from build123d import *

# Parameters (mm, degrees)
SKETCH1_W           = 15
SKETCH1_H           = 49
SKETCH1_R           = 1.6
BOSS_EXTRUDE1_DEPTH = 15
SKETCH2_R           = 2.6
CUT_EXTRUDE1_DEPTH  = 54.394756297
SKETCH5_W           = 15
SKETCH5_H           = 46
BOSS_EXTRUDE3_DEPTH = 10
SKETCH6_R           = 2.6
CUT_EXTRUDE2_DEPTH  = 51.655700568


with BuildPart() as part:
    # Sketch1 → Boss-Extrude1 (new body)
    with BuildSketch(Plane(origin=(0, 0, 0), x_dir=(0, 0, -1), z_dir=(1, 0, 0))):
        with Locations((-7.5, 24.5)):
            Rectangle(SKETCH1_W, SKETCH1_H)
        with Locations((-11, 39.6)):
            Circle(SKETCH1_R, mode=Mode.SUBTRACT)
        with Locations((-11, 9.6)):
            Circle(SKETCH1_R, mode=Mode.SUBTRACT)
    extrude(amount=BOSS_EXTRUDE1_DEPTH)

    # Sketch2 → Cut-Extrude1 (cut, through all)
    with BuildSketch(Plane.XZ):
        with Locations(Location((7.5, 5, 0), (0, 0, 270))):
            Circle(SKETCH2_R)
    extrude(amount=-CUT_EXTRUDE1_DEPTH, mode=Mode.SUBTRACT)

    # Sketch5 → Boss-Extrude3 (add)
    with BuildSketch(Plane(origin=(0, 0, 0), x_dir=(-1, 0, 0), z_dir=(0, 0, -1))):
        with Locations((-7.5, 26)):
            Rectangle(SKETCH5_W, SKETCH5_H)
    extrude(amount=BOSS_EXTRUDE3_DEPTH)

    # Sketch6 → Cut-Extrude2 (cut, through all)
    with BuildSketch(Plane.XZ.offset(-3)):
        with Locations(Location((7.5, -5, 0), (0, 0, 270))):
            Circle(SKETCH6_R)
    extrude(amount=-CUT_EXTRUDE2_DEPTH, mode=Mode.SUBTRACT)


solid = part.part
Can you work these out from the model? Positions are in its coordinate system, mm. A direction names the side the tool comes from. Round coordinates to 2 decimals unless told otherwise and drop trailing zeros. Loops run counter-clockwise (first coordinate to the right, second up) from the corner with the lowest first, then second, coordinate; pieces in that order, holes last. Notation, with made-up numbers: (28.5, 6.5) - (69.5, 6.5) arc R24 ccw to (69.5, 43.5) - close; hole circle Ø1 at (23.5, 60.25). An arc over 180 degrees is marked (long way). Use CSV: the item, a comma, the result in double quotes. Start each with the question number.
1) If we section it at B-B on z = 11: Write out the boundary of the cut face in (x, y).
2) For pin 1 Ø3 at (x, z) = (9, -7.5) entering from -Y; pin 2 Ø2.5 at (x, y) = (8.5, 1) entering from -Z, each with a flat end and sliding along its axis, tell me the tip position at first contact or that it passes through.
3) If we section it at C-C on y = 39.6: Write out the boundary of the cut face in (x, z).
4) If we section it at A-A on x = 7.5: Write out the boundary of the cut face in (y, z), plus the area to 3 significant figures.
5) We'd pull the mould along Y, two halves only. Please class faces 3 (the cylindrical face through (7.395, 41.186, 11.208)), 4 (the flat face through (7, 0, 8)), 5 (the flat face through (8, 26, -10)): released by +Y, released by -Y, zero draft, split by the parting line, or undercut.
6) Please list where these lines run through material, in increasing order: probe 1 along Y at (x, z) = (8.5, 11); probe 2 along Z at (x, y) = (5.75, 41); probe 3 along Z at (x, y) = (9.5, 23.5). Write a range as [from, to].
7) For faces 1 (the flat face through (7, 1, 0)), 2 (the cylindrical face through (5.193, 24.157, 3.8)), which set-ups out of +Z, -Z, +X, -X, +Y, -Y let a thin tool reach every point of the face, with its end or its side?
8) If we section it at D-D on z = -5: Write out the boundary of the cut face in (x, y).
Geometry results:
1,outline,"(0, 0) - (15, 0) - (15, 8) - (0, 8) - close; (0, 11.2) - (15, 11.2) - (15, 38) - (0, 38) - close; (0, 41.2) - (15, 41.2) - (15, 49) - (0, 49) - close"
2,pin 1,"stops at y = 3"
2,pin 2,"stops at z = 0"
3,outline,"(0, -10) - (15, -10) - (15, 9.4) - (0, 9.4) - close; (0, 12.6) - (15, 12.6) - (15, 15) - (0, 15) - close; hole circle Ø5.2 at (7.5, -5); hole circle Ø5.2 at (7.5, 5)"
4,outline,"(0, 0) - (3, 0) - (3, -2.4) - (49, -2.4) - (49, 2.4) - (0, 2.4) - close; (0, 7.6) - (49, 7.6) - (49, 15) - (0, 15) - close; (3, -10) - (49, -10) - (49, -7.6) - (3, -7.6) - close; hole circle Ø3.2 at (9.6, 11); hole circle Ø3.2 at (39.6, 11)"
4,area,"685 mm2"
5,face 3,"undercut"
5,face 4,"released by -Y"
5,face 5,"zero draft"
6,probe 1,"y = [0, 8], [11.2, 38], [41.2, 49]"
6,probe 2,"z = [-10, -6.92], [-3.08, 3.08], [6.92, 10.23], [11.77, 15]"
6,probe 3,"z = [-10, -6.66], [-3.34, 3.34], [6.66, 15]"
7,face 1,"-Z, +X, -X, -Y"
7,face 2,"+Y, -Y"
8,outline,"(0, 3) - (4.9, 3) - (4.9, 49) - (0, 49) - close; (10.1, 3) - (15, 3) - (15, 49) - (10.1, 49) - close"
